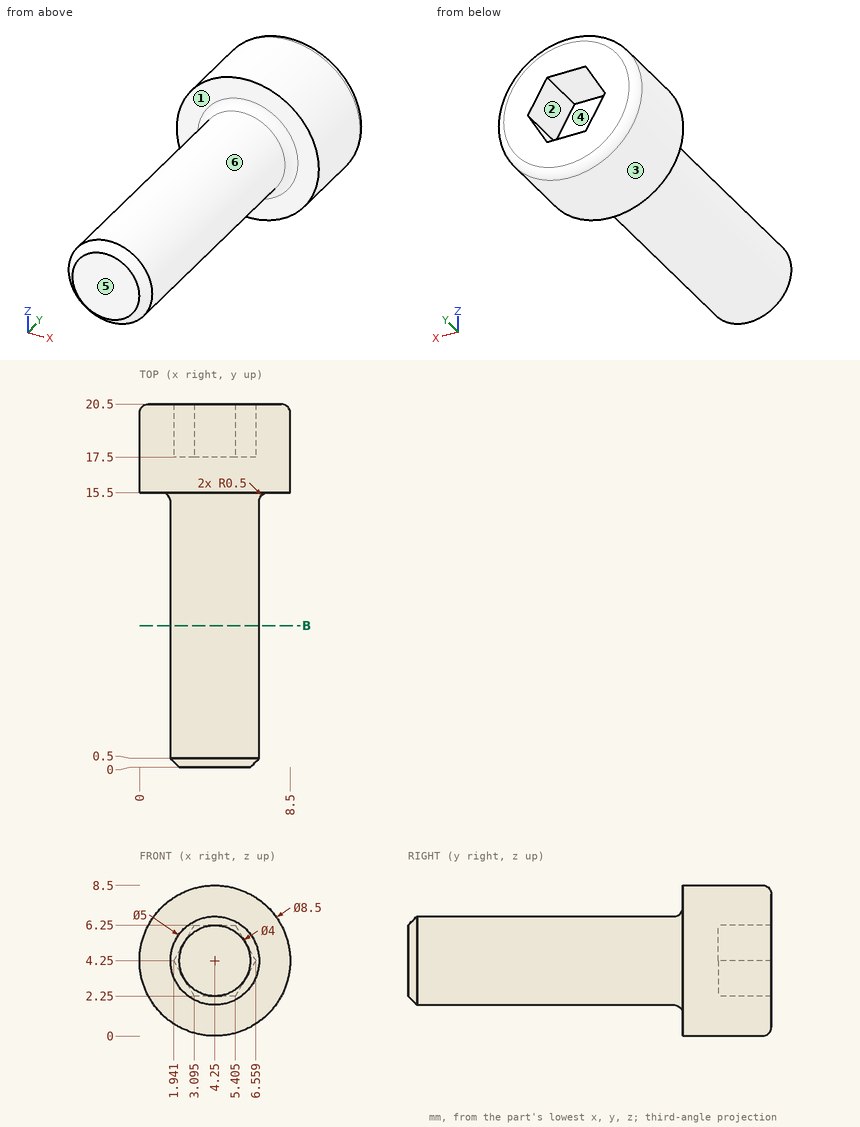
Here's the drawing with two shaded views (mm, measured from the low corner). I have some questions. A direction names the side the tool comes from. Give positions to 0.01 mm unless a question says otherwise; leave off trailing zeros. Loops run counter-clockwise (first coordinate to the right, second up) from the corner with the lowest first, then second, coordinate; pieces in that order, holes last. Notation, with made-up numbers: (-28.5, 80) -> (15.5, 80) arc R17 cw to (15.5, 111) -> close; hole circle Ø8 at (82, -2.5). An arc over 180 degrees is marked (long way). One line per item, written item: value.
Q1. On a 3-axis mill with a long thin cutter (end or side, diameter ignored), from which of +Z, -Z, +X, -X, +Y, -Y can I reach the whole of each face in a straight line? I mean the marked faces 1, 2 and 3. Say none if no direction works.
Answers follow:
face 1: -Y
face 2: +Y
face 3: +Y, -Y
Q2. We'd pull the mould along Z, two halves only. Please class the marked faces 4, 5 and 6: pulls with the +Z half, pulls with the -Z half, needs draft (parallel to the pull), parting line crosses it, or undercut.
Answers follow:
face 4: undercut
face 5: needs draft
face 6: parting line crosses it
Q3. I'm going to push flat-ended pins straight in: pin 1 Ø3 at (x, y) = (6.5, 4.5) entering from +Z (1 decimal); pin 2 Ø1.2 at (x, z) = (5, 5) entering from +Y; pin 3 Ø1 at (x, y) = (5, 16.5) entering from -Z. Where does each tip first touch, or does it pass through?
Answers follow:
pin 1: z = 6.6
pin 2: y = 17.5
pin 3: z = 0.01
Q4. Suppose I cut it at B-B on y = 8. Please give me the cut outline in (x, z).
Answers follow:
outline: circle Ø5 at (4.25, 4.25)
Q5. If I drill on line 1 along Y through (x, z) = (7.5, 6); line 2 along X through (y, z) = (19, 5) (1 decimal); line 3 along X through (y, z) = (18.5, 4.5) (1 decimal), over which ranges is the centre line in solid material (lowest first)?
Answers follow:
line 1: 15.5 to 20.5
line 2: 0.1 to 2.4, 6.1 to 8.4
line 3: 0 to 2.1, 6.4 to 8.5
